Geometry: final body of the model. Coordinates: model frame, mm. Give positions to 0.01 mm unless a question says otherwise; leave off trailing zeros. Write each loop counter-clockwise with the first axis right and the second up, starting at its lowest first coordinate (ties: lowest second). Pieces come first, ordered by that corner, then holes.
Q1. Pin query (flat end, axial travel): pin 1 Ø3 at (y, z) = (-2.5, 105.5) entering from +X. Return the tip coordinate at first contact, or that it passes through.
Q2. Line query: line 1 (X direction, y = 1.25, z = 41); line 2 (Y direction, x = -1.75, z = 89); line 3 (Y direction, x = -2.5, z = -126). Output: solid intervals per line, ascending.
Q3. Section A-A (z = -15). Return the cut outline in (x, y) (3 decimals), plus the area to 3 significant figures.
from build123d import *

# Parameters (mm, degrees)
BOSS_EXTRUDE1_DEPTH = 150
FILLET1_R           = 0.2


with BuildPart() as part:
    # Sketch1 → Boss-Extrude1 (new, symmetric)
    with BuildSketch(Plane.XY):
        Polygon((3.666174209, 0), (1.833087105, 3.175), (-1.833087105, 3.175), (-3.666174209, 0), (-1.833087105, -3.175), (1.833087105, -3.175), align=None)
    extrude(amount=BOSS_EXTRUDE1_DEPTH, both=True)

    # Fillet1
    fillet1_edges = [part.edges().sort_by_distance(p)[0] for p in [
        (1.833087105, -3.175, 0),
        (-1.833087105, -3.175, 0),
        (-3.666174209, 0, 0),
        (-1.833087105, 3.175, 0),
        (1.833087105, 3.175, 0),
        (3.666174209, 0, 0),
        (0, 3.175, 150),
        (-2.749630657, 1.5875, 150),
        (-2.749630657, -1.5875, 150),
        (0, -3.175, 150),
        (2.749630657, -1.5875, 150),
        (0, -3.175, -150),
        (-2.749630657, -1.5875, -150),
        (-2.749630657, 1.5875, -150),
        (0, 3.175, -150),
        (2.749630657, 1.5875, -150),
        (2.749630657, -1.5875, -150),
        (2.749630657, 1.5875, 150),
    ]]
    fillet(fillet1_edges, radius=FILLET1_R)


solid = part.part
Computed:
1. pin 1: stops at x = 3.09
2. line 1: x = -2.94 to 2.94
2. line 2: y = -3.17 to 3.17
2. line 3: y = -2.02 to 2.02
3. outline: (-3.608, -0.1) - (-1.891, -3.075) arc R0.2 ccw to (-1.718, -3.175) - (1.718, -3.175) arc R0.2 ccw to (1.891, -3.075) - (3.608, -0.1) arc R0.2 ccw to (3.608, 0.1) - (1.891, 3.075) arc R0.2 ccw to (1.718, 3.175) - (-1.718, 3.175) arc R0.2 ccw to (-1.891, 3.075) - (-3.608, 0.1) arc R0.2 ccw to start
3. area: 34.9 mm2
